```python
from build123d import *

# Parameters (mm, degrees)
ESQUISSE1_R        = 2
ESQUISSE1_R_2      = 7.5
ESQUISSE1_R_3      = 2.5
BOSS_EXTRU_1_DEPTH = 6


with BuildPart() as part:
    # Esquisse1 → Boss.-Extru.1 (new body)
    with BuildSketch(Plane(origin=(0, 0, 0), x_dir=(1, 0, 0), z_dir=(0, 1, 0))):
        with BuildLine():
            Line((-74.229814571, -3.895021171), (-74.229814571, 3.895021171))
            ThreePointArc((-74.229814571, 3.895021171), (-72.17956204, 8.844768639), (-67.229814571, 10.895021171))
            Line((-67.229814571, 10.895021171), (-9.309179879, 10.895021171))
            ThreePointArc((-9.309179879, 10.895021171), (-5.848907465, 11.810079526), (-3.293306817, 14.316016937))
            ThreePointArc((-3.293306817, 14.316016937), (48.770185429, 0), (-3.293306817, -14.316016937))
            ThreePointArc((-3.293306817, -14.316016937), (-5.848907465, -11.810079526), (-9.309179879, -10.895021171))
            Line((-9.309179879, -10.895021171), (-67.229814571, -10.895021171))
            ThreePointArc((-67.229814571, -10.895021171), (-72.17956204, -8.844768639), (-74.229814571, -3.895021171))
        make_face()
        with Locations((40.770185429, 0)):
            Circle(ESQUISSE1_R, mode=Mode.SUBTRACT)
        with Locations((20.770185429, 0)):
            Circle(ESQUISSE1_R_2, mode=Mode.SUBTRACT)
        with Locations((0.770185429, 0)):
            Circle(ESQUISSE1_R, mode=Mode.SUBTRACT)
        with Locations((-39.229814571, 0)):
            Circle(ESQUISSE1_R_3, mode=Mode.SUBTRACT)
    extrude(amount=BOSS_EXTRU_1_DEPTH)


solid = part.part
```
Part model, mm, in its own coordinate system. A direction names the side the tool comes from. Give positions to 0.01 mm unless a question says otherwise; leave off trailing zeros. Order: outer loops, then holes, each group sorted by start corner. A loop starts at its lowest first (then second) coordinate and runs counter-clockwise, first axis right, second up. Notation, with made-up numbers: (79, 5.5) - (102, 5.5) arc R29 cw to (102, 27.5) - close; hole circle Ø2 at (40, 67). An arc over 180 degrees is marked (long way). Use one line per item in the form item = value.
Item 1: Two-plate mould, pull along Z, no slides. Class faces 3 (the face through (-5.893, 2.958, -11.785)), 4 (the face through (-74.23, 3, 0)), 5 (the face through (-38, 3, 10.895)), 6 (the face through (19.14, 2.96, 7.32)): released by +Z, released by -Z, zero draft, split by the parting line, or undercut.
Solution:
face_3 = released by -Z
face_4 = zero draft
face_5 = released by +Z
face_6 = undercut
Item 2: Slice it at B-B on x = 1. Give the cut face in (y, z).
Solution:
outline = (0, -19.83) - (6, -19.83) - (6, -1.99) - (0, -1.99) - close; (0, 1.99) - (6, 1.99) - (6, 19.83) - (0, 19.83) - close
Item 3: Slice it at D-D on z = 20. Give the cut face in (x, y).
Solution:
outline = (1.17, 0) - (40.37, 0) - (40.37, 6) - (1.17, 6) - close
Item 4: Slice it at C-C on x = -29.5. Give the cut face in (y, z).
Solution:
outline = (0, -10.9) - (6, -10.9) - (6, 10.9) - (0, 10.9) - close
Item 5: Which spindle directions (+Z, -Z, +X, -X, +Y, -Y) get a long thin tool onto all of the face, cutting with end or side? Do faces 1 (the face through (-72.125, 2.958, 8.899)), 2 (the face through (-39, 3, -10.895)). Say none if no direction does.
Solution:
face_1 = +Z, -X, +Y, -Y
face_2 = -Z, -X, +Y, -Y
Item 6: Slice it at A-A on z = 0. Give the cut face in (x, y).
Solution:
outline = (-74.23, 0) - (-41.73, 0) - (-41.73, 6) - (-74.23, 6) - close; (-36.73, 0) - (-1.23, 0) - (-1.23, 6) - (-36.73, 6) - close; (2.77, 0) - (13.27, 0) - (13.27, 6) - (2.77, 6) - close; (28.27, 0) - (38.77, 0) - (38.77, 6) - (28.27, 6) - close; (42.77, 0) - (48.77, 0) - (48.77, 6) - (42.77, 6) - close
Item 7: Probe probe 1 along X at (y, z) = (4.65, 0); probe 2 along Z at (x, y) = (-29, 3.25); probe 3 along Z at (x, y) = (-39, 2.8). List the from-to ranges inside material, lowest first. Write a range as from..to.
Solution:
probe_1 = -74.23..-41.73, -36.73..-1.23, 2.77..13.27, 28.27..38.77, 42.77..48.77
probe_2 = -10.9..10.9
probe_3 = -10.9..-2.49, 2.49..10.9
Item 8: Pin check, flat tips, straight feed: pin 1 Ø3 at (x, y) = (-48, 3.5) entering from +Z (3 decimals); pin 2 Ø3 at (y, z) = (1.5, -15.5) entering from +X; pin 3 Ø1 at (x, y) = (-39.5, 4.5) entering from -Z (3 decimals). Stop position of each tip, or through.
Solution:
pin_1 = 10.895
pin_2 = 45.02
pin_3 = -10.895
